from build123d import *

# Parameters (mm, degrees)
SKETCH1_W                            = 4.75
SKETCH1_H                            = 7
FILLET1_R                            = 1
SKETCH16_W                           = 16
SKETCH16_H                           = 1
CUT_EXTRUDE5_DEPTH                   = 1
CUT_EXTRUDE5_DIRECTION_2_REACH       = 18.492
CUT_EXTRUDE6_REACH                   = 15.304
SKETCH17_W                           = 3.5
SKETCH17_H                           = 5.261387212
CUT_EXTRUDE7_DEPTH                   = 18.408690359
CUT_EXTRUDE7_DEPTH_BACK              = 18.408690359
SKETCH18_R                           = 1.2
CUT_EXTRUDE10_START                  = -6
SKETCH21_R                           = 0.825
CUT_EXTRUDE10_DEPTH                  = 6
CUT_EXTRUDE11_DEPTH                  = 18.26991621
CUT_EXTRUDE11_DEPTH_BACK             = 18.26991621
SKETCH22_R                           = 1.2
CUT_EXTRUDE9_REACH                   = 20.603
CUT_EXTRUDE9_END_RADIUS              = 8
SKETCH20_R                           = 1.2
CUT_EXTRUDE12_REACH                  = 21.585
SKETCH19_R                           = 2.25
CUT_EXTRUDE13_REACH                  = 21.585
CUT_EXTRUDE13_END_RADIUS             = 8
SKETCH24_R                           = 2.25
CUT_EXTRUDE14_REACH                  = 18.492
CUT_EXTRUDE14_END_RADIUS             = 8
SKETCH25_W                           = 2.25
SKETCH25_H                           = 1
CUT_EXTRUDE14_DIRECTION_2_REACH      = 18.492
CUT_EXTRUDE14_DIRECTION_2_END_RADIUS = 8
M2_5_CLEARANCE_HOLE1_D               = 2.9
M2_5_CLEARANCE_HOLE1_DEPTH           = 7.729752102
M2_5_CLEARANCE_HOLE1_TIP             = 0.871247898
CUT_EXTRUDE15_START                  = -12
SKETCH29_W                           = 4
SKETCH29_H                           = 2.25
CUT_EXTRUDE15_DEPTH                  = 12
FILLET3_R                            = 0.25
SKETCH30_R                           = 8
CUT_EXTRUDE19_DEPTH                  = 1


with BuildPart() as part:
    # Sketch1 → Revolve1 (revolve)
    with BuildSketch(Plane.XY, mode=Mode.PRIVATE) as revolve1_sk:
        with Locations((5.625, 3.5)):
            Rectangle(SKETCH1_W, SKETCH1_H)
    revolve(revolve1_sk.sketch.rotate(Axis((0, 0, 0), (0, 1, 0)), 90), axis=Axis((0, 0, 0), (0, 1, 0)))

    # Sketch1<3> → Revolve2 (revolve)
    with BuildSketch(Plane.XY, mode=Mode.PRIVATE) as revolve2_sk:
        Polygon((0.825, 7), (3.25, 7), (8, 7), (8, 12), (0.825, 12), align=None)
    revolve(revolve2_sk.sketch.rotate(Axis((0, 0, 0), (0, 1, 0)), 90), axis=Axis((0, 0, 0), (0, 1, 0)))

    # Fillet1
    fillet1_edges = [part.edges().sort_by_distance(p)[0] for p in [
        (0, 12, 8),
    ]]
    fillet(fillet1_edges, radius=FILLET1_R)

    # Sketch16 → Cut-Extrude5 (cut)
    with BuildSketch(Plane.XY):
        with Locations((0, 5.5)):
            Rectangle(SKETCH16_W, SKETCH16_H)
    extrude(amount=-CUT_EXTRUDE5_DEPTH, mode=Mode.SUBTRACT)

    # Sketch16 → Cut-Extrude5 direction 2 (cut, up to next)
    with BuildSketch(Plane.XY, mode=Mode.PRIVATE) as cut_extrude5_direction_2_sk1:
        with Locations((0, 5.5)):
            Rectangle(SKETCH16_W, SKETCH16_H)
    cut_extrude5_direction_2_tool1 = extrude(cut_extrude5_direction_2_sk1.sketch, amount=CUT_EXTRUDE5_DIRECTION_2_REACH, mode=Mode.PRIVATE) & part.part
    add(cut_extrude5_direction_2_tool1.solids().sort_by_distance((0, 5.5, 0))[0], mode=Mode.SUBTRACT)

    # Sketch17 → Cut-Extrude6 (cut, up to next)
    with BuildSketch(Plane(origin=(0, 5, 0), x_dir=(1, 0, 0), z_dir=(0, 1, 0)), mode=Mode.PRIVATE) as cut_extrude6_sk1:
        with Locations((0, -5.369306394)):
            Rectangle(SKETCH17_W, SKETCH17_H)
    cut_extrude6_tool1 = extrude(cut_extrude6_sk1.sketch, amount=-CUT_EXTRUDE6_REACH, mode=Mode.PRIVATE) & part.part
    add(cut_extrude6_tool1.solids().sort_by_distance((0, 5, 5.369306))[0], mode=Mode.SUBTRACT)

    # Sketch18 → Cut-Extrude7 (cut, two sides: drawn at the far end of the back side and taken through both)
    with BuildSketch(Plane.ZY.offset(-1.75).offset(-CUT_EXTRUDE7_DEPTH_BACK)):
        with Locations((4.772430143, 2.5)):
            Circle(SKETCH18_R)
    extrude(amount=CUT_EXTRUDE7_DEPTH + CUT_EXTRUDE7_DEPTH_BACK, mode=Mode.SUBTRACT)

    # Sketch21 → Cut-Extrude10 (cut)
    with BuildSketch(Plane(origin=(0, 12, 0), x_dir=(1, 0, 0), z_dir=(0, 1, 0)).offset(CUT_EXTRUDE10_START)):
        Circle(SKETCH21_R)
        Polygon((-1.5, -1.6), (-1.5, -11.891029443), (1.5, -11.891029443), (1.5, -1.6), (0.566237583, -1.6), (0.566237583, -0.6), (-0.566237583, -0.6), (-0.566237583, -1.6), align=None)
    extrude(amount=CUT_EXTRUDE10_DEPTH, mode=Mode.SUBTRACT)

    # Sketch22 → Cut-Extrude11 (cut, two sides: drawn at the far end of the back side and taken through both)
    with BuildSketch(Plane(origin=(-1.5, 0, 0), x_dir=(0, 0, -1), z_dir=(1, 0, 0)).offset(-CUT_EXTRUDE11_DEPTH_BACK)):
        with Locations((-3.358116823, 8.5)):
            Circle(SKETCH22_R)
    extrude(amount=CUT_EXTRUDE11_DEPTH + CUT_EXTRUDE11_DEPTH_BACK, mode=Mode.SUBTRACT)

    # Cut-Extrude9: up to this cylinder (the profile starts inside it)
    cut_extrude9_end = Plane(origin=(0, 5.9847245, 0), z_dir=(0, -1, 0)) * Cylinder(CUT_EXTRUDE9_END_RADIUS, 65.175449, mode=Mode.PRIVATE)
    # Sketch20 → Cut-Extrude9 (cut, up to the surface)
    with BuildSketch(Plane(origin=(-3.75, 0, 0), x_dir=(0, 0, -1), z_dir=(1, 0, 0)), mode=Mode.PRIVATE) as cut_extrude9_sk1:
        Polygon((-2.463029066, 2.5), (-3.617729604, 4.5), (-5.927130681, 4.5), (-7.08183122, 2.5), (-5.927130681, 0.5), (-3.617729604, 0.5), align=None)
    cut_extrude9_tool1 = extrude(cut_extrude9_sk1.sketch, amount=-CUT_EXTRUDE9_REACH, mode=Mode.PRIVATE) & cut_extrude9_end
    add(cut_extrude9_tool1.solids().sort_by_distance((-3.75, 2.5, 4.77243))[0], mode=Mode.SUBTRACT)
    # Sketch20 → Cut-Extrude9 (cut, up to the surface)
    with BuildSketch(Plane(origin=(-3.75, 0, 0), x_dir=(0, 0, -1), z_dir=(1, 0, 0)), mode=Mode.PRIVATE) as cut_extrude9_sk2:
        Polygon((-1.048715746, 8.5), (-2.203416284, 10.5), (-4.512817361, 10.5), (-5.6675179, 8.5), (-4.512817361, 6.5), (-2.203416284, 6.5), align=None)
        with Locations((-3.358116823, 8.5)):
            Circle(SKETCH20_R, mode=Mode.SUBTRACT)
    cut_extrude9_tool2 = extrude(cut_extrude9_sk2.sketch, amount=-CUT_EXTRUDE9_REACH, mode=Mode.PRIVATE) & cut_extrude9_end
    add(cut_extrude9_tool2.solids().sort_by_distance((-3.75, 9.469449, 1.678981))[0], mode=Mode.SUBTRACT)

    # Sketch19 → Cut-Extrude12 (cut, up to next)
    with BuildSketch(Plane.ZY.offset(-5.25), mode=Mode.PRIVATE) as cut_extrude12_sk1:
        with Locations((4.772430143, 2.5)):
            Circle(SKETCH19_R)
    cut_extrude12_tool1 = extrude(cut_extrude12_sk1.sketch, amount=-CUT_EXTRUDE12_REACH, mode=Mode.PRIVATE) & part.part
    add(cut_extrude12_tool1.solids().sort_by_distance((5.25, 2.5, 4.77243))[0], mode=Mode.SUBTRACT)

    # Cut-Extrude13: up to this cylinder (the profile starts inside it)
    cut_extrude13_end = Plane(origin=(0, 8.5, 0), z_dir=(0, -1, 0)) * Cylinder(CUT_EXTRUDE13_END_RADIUS, 60.17, mode=Mode.PRIVATE)
    # Sketch24 → Cut-Extrude13 (cut, up to the surface)
    with BuildSketch(Plane.ZY.offset(-5.25), mode=Mode.PRIVATE) as cut_extrude13_sk1:
        with Locations((3.358116823, 8.5)):
            Circle(SKETCH24_R)
    cut_extrude13_tool1 = extrude(cut_extrude13_sk1.sketch, amount=-CUT_EXTRUDE13_REACH, mode=Mode.PRIVATE) & cut_extrude13_end
    add(cut_extrude13_tool1.solids().sort_by_distance((5.25, 8.5, 3.358117))[0], mode=Mode.SUBTRACT)

    # Cut-Extrude14: up to this cylinder (the profile starts inside it)
    cut_extrude14_end = Plane(origin=(0, 5.5, 0), z_dir=(0, -1, 0)) * Cylinder(CUT_EXTRUDE14_END_RADIUS, 53.984, mode=Mode.PRIVATE)
    # Sketch25 → Cut-Extrude14 (cut, up to the surface)
    with BuildSketch(Plane.ZY, mode=Mode.PRIVATE) as cut_extrude14_sk1:
        with Locations((-2.125, 5.5)):
            Rectangle(SKETCH25_W, SKETCH25_H)
    cut_extrude14_tool1 = extrude(cut_extrude14_sk1.sketch, amount=-CUT_EXTRUDE14_REACH, mode=Mode.PRIVATE) & cut_extrude14_end
    add(cut_extrude14_tool1.solids().sort_by_distance((0, 5.5, -2.125))[0], mode=Mode.SUBTRACT)

    # Cut-Extrude14 direction 2: up to this cylinder (the profile starts inside it)
    cut_extrude14_direction_2_end = Plane(origin=(0, 5.5, 0), z_dir=(0, -1, 0)) * Cylinder(CUT_EXTRUDE14_DIRECTION_2_END_RADIUS, 53.984, mode=Mode.PRIVATE)
    # Sketch25 → Cut-Extrude14 direction 2 (cut, up to the surface)
    with BuildSketch(Plane.ZY, mode=Mode.PRIVATE) as cut_extrude14_direction_2_sk1:
        with Locations((-2.125, 5.5)):
            Rectangle(SKETCH25_W, SKETCH25_H)
    cut_extrude14_direction_2_tool1 = extrude(cut_extrude14_direction_2_sk1.sketch, amount=CUT_EXTRUDE14_DIRECTION_2_REACH, mode=Mode.PRIVATE) & cut_extrude14_direction_2_end
    add(cut_extrude14_direction_2_tool1.solids().sort_by_distance((0, 5.5, -2.125))[0], mode=Mode.SUBTRACT)

    # M2.5 Clearance Hole1
    with Locations(Plane(origin=(0, 0, -8), x_dir=(-1, 0, 0), z_dir=(0, 0, -1))):
        with Locations((0, 8.5), (0, 2.5)):
            Hole(M2_5_CLEARANCE_HOLE1_D / 2, depth=M2_5_CLEARANCE_HOLE1_DEPTH)
            with Locations((0, 0, -(M2_5_CLEARANCE_HOLE1_DEPTH + M2_5_CLEARANCE_HOLE1_TIP / 2))):  # 118° drill point
                Cone(0, M2_5_CLEARANCE_HOLE1_D / 2, M2_5_CLEARANCE_HOLE1_TIP, mode=Mode.SUBTRACT)

    # Sketch29 → Cut-Extrude15 (cut)
    with BuildSketch(Plane(origin=(0, 12, 0), x_dir=(1, 0, 0), z_dir=(0, 1, 0)).offset(CUT_EXTRUDE15_START)):
        with Locations((0, 5.5)):
            Rectangle(SKETCH29_W, SKETCH29_H)
    extrude(amount=CUT_EXTRUDE15_DEPTH, mode=Mode.SUBTRACT)

    # Fillet3
    fillet3_edges = [part.edges().sort_by_distance(p)[0] for p in [
        (0.566237583, 9.5, 1.6),
        (-0.566237583, 9.5, 1.6),
    ]]
    fillet(fillet3_edges, radius=FILLET3_R)

    # Sketch30 → Cut-Extrude19 (cut)
    with BuildSketch(Plane(origin=(0, 12, 0), x_dir=(1, 0, 0), z_dir=(0, 1, 0))):
        Circle(SKETCH30_R)
    extrude(amount=-CUT_EXTRUDE19_DEPTH, mode=Mode.SUBTRACT)


solid = part.part
The model under review builds one solid part; all positions refer to its coordinate system, in mm. A direction names the side the tool comes from. Give positions to 0.01 mm unless a question says otherwise; leave off trailing zeros. Order: outer loops, then holes, each group sorted by start corner. A loop starts at its lowest first (then second) coordinate and runs counter-clockwise, first axis right, second up. Notation, with made-up numbers: (-19, -1.75) -> (-14, -1.75) arc R21 cw to (-14, 2.25) -> close; hole circle Ø4 at (1.25, 38). An arc over 180 degrees is marked (long way). Write item = value, one per line. Start each with the question number.
(1) For L1, parallel to Y at x = -4.25, z = -3; L2, parallel to Y at x = 3.75, z = 5.5; L3, parallel to X at y = 8, z = 5.25, list the stretches that pass through material, from the lowest coordinate up. Write a range as from..to.
(2) Take a section at B-B (x = 4.25). Write out the cut boundary in (y, z).
(3) Draft analysis for pull direction Y (two halves, no side actions). For faces 5 (the flat face through (1.75, 2.5, 6.4)), 6 (the flat face through (-5, 6, 2)), 7 (the flat face through (2, 11, 0)), 8 (the flat face through (-1, 7, -1)), state which applies: +Y half, -Y half, draft (parallel to the pull), parting line (faces both ways), or undercut.
(4) Take a section at C-C (z = -3.5). Write out the cut boundary in (x, y), plus the area to 3 significant figures.
(5) Take a section at D-D (y = 9). State how many separate pieces and enclosed holes the cut face has, plus the area to 3 significant figures.
(6) For pin 1 Ø1.9 at (y, z) = (8.5, 3.36) entering from -X; pin 2 Ø5 at (x, y) = (4.5, 1.5) entering from +Z; pin 3 Ø0.7 at (y, z) = (3, -5.5) entering from +X; pin 4 Ø3 at (y, z) = (2.5, 4.77) entering from +X, all flat-tipped, find the tip position at first contact; note any pin that passes through.
(7) Take a section at A-A (x = -2.75). Write out the cut boundary in (y, z).
(8) Tool access review of faces 1 (the flat face through (-2, 5, -5)), 2 (the flat face through (-5, 4.5, 4)), 3 (the cylindrical face through (-1.45, 8.56, -7.3)), 4 (the flat face through (5, 6, 1)): name each direction out of +Z, -Z, +X, -X, +Y, -Y from which nothing blocks a thin tool from reaching the whole face with its end or side.
Returned:
q1.L1 = 0..5, 6..11
q1.L2 = 0..1.55, 3.45..5, 6..11
q1.L3 = -3.75..-1.5, 1.5..5.25
q2.outline = (0, -6.78) -> (11, -6.78) -> (11, 6.78) -> (6, 6.78) -> (6, -3.25) -> (5, -3.25) -> (5, 6.78) -> (0, 6.78) -> close; hole circle Ø2.4 at (2.5, 4.77); hole circle Ø2.4 at (8.5, 3.36)
q3.face_5 = draft
q3.face_6 = undercut
q3.face_7 = +Y half
q3.face_8 = -Y half
q4.outline = (-7.19, 0) -> (7.19, 0) -> (7.19, 11) -> (-7.19, 11) -> close; hole circle Ø2.9 at (0, 2.5); hole circle Ø2.9 at (0, 8.5)
q4.area = 145 mm²
q5.separate_pieces = 4
q5.enclosed_holes = 0
q5.area = 121 mm²
q6.pin_1 = through
q6.pin_2 = 7.75
q6.pin_3 = 6.12
q6.pin_4 = 5.25
q7.outline = (0, -7.51) -> (11, -7.51) -> (11, 7.51) -> (6, 7.51) -> (6, 1.73) -> (7, 1.73) -> (7, -1.73) -> (6, -1.73) -> (6, -3.25) -> (5, -3.25) -> (5, -1.73) -> (0, -1.73) -> close; (0, 1.73) -> (5, 1.73) -> (5, 7.51) -> (0, 7.51) -> close; hole circle Ø2.4 at (2.5, 4.77); hole circle Ø2.4 at (8.5, 3.36)
q8.face_1 = +Y, -Y
q8.face_2 = -X
q8.face_3 = -Z
q8.face_4 = +Z, +X, -X
